```python
from build123d import *

# Parameters (mm, degrees)
SKETCH1_R             = 2.6
SKETCH1_R_2           = 5.1
BASE_FLANGE1_DEPTH    = 2
M5X0_8_TAPPED_HOLE1_D = 4.2


# Sheet-metal steps are written as plain solids
with BuildPart() as part:
    # Sketch1 → Base-Flange1 (new body)
    with BuildSketch(Plane.XY):
        with BuildLine():
            Line((-35, 15), (-35, -10))
            ThreePointArc((-35, -10), (-33.535533906, -13.535533906), (-30, -15))
            Line((-30, -15), (30, -15))
            ThreePointArc((30, -15), (33.535533906, -13.535533906), (35, -10))
            Line((35, -10), (35, 15))
            ThreePointArc((35, 15), (33.535533906, 18.535533906), (30, 20))
            Line((30, 20), (7.5, 20))
            ThreePointArc((7.5, 20), (6.792893219, 20.292893219), (6.5, 21))
            Line((6.5, 21), (6.5, 58))
            ThreePointArc((6.5, 58), (0, 64.5), (-6.5, 58))
            Line((-6.5, 58), (-6.5, 21))
            ThreePointArc((-6.5, 21), (-6.792893219, 20.292893219), (-7.5, 20))
            Line((-7.5, 20), (-30, 20))
            ThreePointArc((-30, 20), (-33.535533906, 18.535533906), (-35, 15))
        make_face()
        with Locations((-20, 0)):
            Circle(SKETCH1_R, mode=Mode.SUBTRACT)
        Circle(SKETCH1_R_2, mode=Mode.SUBTRACT)
        with Locations((20, 0)):
            Circle(SKETCH1_R, mode=Mode.SUBTRACT)
    extrude(amount=-BASE_FLANGE1_DEPTH)

    # M5x0.8 Tapped Hole1 (through all)
    with Locations(Plane.XY):
        with Locations((0, 58)):
            Hole(M5X0_8_TAPPED_HOLE1_D / 2)


solid = part.part
```
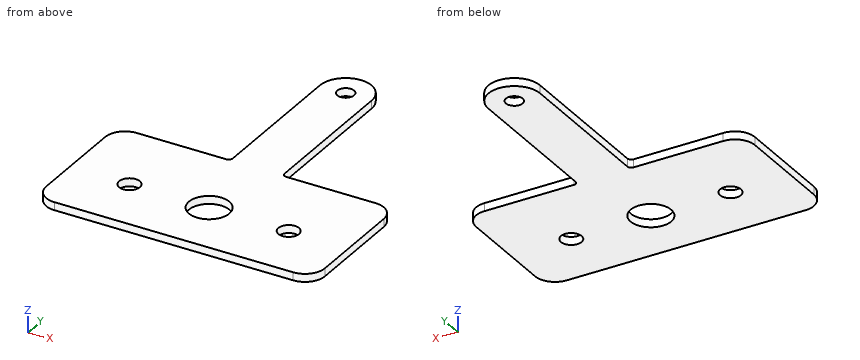
Could you check a few things on this model? Use its own coordinates, in mm. Coordinates: 2 decimals unless noted, no trailing zeros. Loops run counter-clockwise (first coordinate to the right, second up) from the corner with the lowest first, then second, coordinate; pieces in that order, holes last. Notation, with made-up numbers: M 36,23 L 92,23 A35 ccw 92,59 Z; hole C 19,10.5 d6. An arc over 180 degrees is marked long. Put each result on its own line as item: value. Start each with the question number.
(1) Suppose I cut it at D-D on x = 0. Please give me the cut outline in (y, z), then the cut area to 3 significant figures.
(2) Suppose I cut it at C-C on y = 0. Please give me the cut outline in (x, z).
(3) Will these pins go through, and if not, where does the flat tip stop? P1, Ø13.5, axis at x = 0, y = 0, coming from the +Z side; P2, Ø1, axis at y = 46, z = -1, coming from the +X side.
(4) Suppose I cut it at A-A on x = -20. Please give me the cut outline in (y, z).
(5) I need wall thicknesses on line 1 (Y direction, x = 0, z = -1.35); line 2 (Y direction, x = -20, z = -1.1); line 3 (Y direction, x = -0.5, z = -1.05). Which ranges of each line are inside material? Lowest first, please. Write a range as from..to.
(6) Suppose I cut it at B-B on z = -0.9. Please give me the cut outline in (x, y).
Solutions:
1. outline: M -15,-2 L -5.1,-2 L -5.1,0 L -15,0 Z; M 5.1,-2 L 55.9,-2 L 55.9,0 L 5.1,0 Z; M 60.1,-2 L 64.5,-2 L 64.5,0 L 60.1,0 Z
1. area: 130 mm2
2. outline: M -35,-2 L -22.6,-2 L -22.6,0 L -35,0 Z; M -17.4,-2 L -5.1,-2 L -5.1,0 L -17.4,0 Z; M 5.1,-2 L 17.4,-2 L 17.4,0 L 5.1,0 Z; M 22.6,-2 L 35,-2 L 35,0 L 22.6,0 Z
3. P1: stops at z = 0
3. P2: stops at x = 6.5
4. outline: M -15,-2 L -2.6,-2 L -2.6,0 L -15,0 Z; M 2.6,-2 L 20,-2 L 20,0 L 2.6,0 Z
5. line 1: y = -15..-5.1, 5.1..55.9, 60.1..64.5
5. line 2: y = -15..-2.6, 2.6..20
5. line 3: y = -15..-5.08, 5.08..55.96, 60.04..64.48
6. outline: M -35,-10 A5 ccw -30,-15 L 30,-15 A5 ccw 35,-10 L 35,15 A5 ccw 30,20 L 7.5,20 A1 cw 6.5,21 L 6.5,58 A6.5 ccw -6.5,58 L -6.5,21 A1 cw -7.5,20 L -30,20 A5 ccw -35,15 Z; hole C -20,0 d5.2; hole C 0,0 d10.2; hole C 0,58 d4.2; hole C 20,0 d5.2
